Could you check a few things on this model? Use its own coordinates, in mm. A direction names the side the tool comes from. Round coordinates to 2 decimals unless told otherwise and drop trailing zeros. Write each loop counter-clockwise with the first axis right and the second up, starting at its lowest first coordinate (ties: lowest second). Pieces come first, ordered by that corner, then holes. Notation, with made-up numbers: (12.5, 49) -> (41.5, 49) arc R19 cw to (41.5, 67) -> close; hole circle Ø8 at (7.25, 71.25). An arc over 180 degrees is marked (long way). Answer as CSV lines item,"result". Start each with the question number.
Q1. Will these pins go through, and if not, where does the flat tip stop? pin 1 Ø3 at (x, y) = (-23, 2) entering from -Z; pin 2 Ø6 at (x, y) = (-25, 24.5) entering from +Z.
Q2. Imagine slicing it at B-B on z = 42. Please give me the cut outline in (x, y), and give its area (3 significant figures).
Q3. Imagine slicing it at C-C on y = 38. Please give me the cut outline in (x, z).
Q4. If I drill on line 1 (X direction, y = 42, z = 45.5); line 2 (Y direction, x = -59, z = 18); line 3 (Z direction, x = -51.5, y = 20), over which ranges is the centre line in solid material (lowest first)? Write a range as [from, to].
Q5. Imagine slicing it at D-D on y = 16.5. Please give me the cut outline in (x, z).
Q6. If we mould it in two halves opening along X, with no side actions, what happens to faces 1 (the flat face through (-73.66, 16, 19)), 2 (the flat face through (-37, 61.133, 25)), 3 (the flat face through (-37, -11.209, 27))? For each: pulls with the +X half, pulls with the -X half, needs draft (parallel to the pull), parting line crosses it, or undercut.
Q7. Imagine slicing it at A-A on x = -33. Please give me the cut outline in (y, z), and give its area (3 significant figures).
Q8. For faces 4 (the flat face through (-72.493, 24, 16)), 5 (the cylindrical face through (-0.7, 25.75, 43.85)), which set-ups out of +Z, -Z, +X, -X, +Y, -Y let a thin tool reach every point of the face, with its end or its side?
from build123d import *

# Parameters (mm, degrees)
F0_W     = 73.66
F0_H     = 73.66
F1_DEPTH = 50.8
F2_W     = 71.12
F2_H     = 71.12
F3_DEPTH = 48.26
F4_R     = 12.7
F5_DEPTH = 87.376


with BuildPart() as f1:
    # F0 (on Top) → F1 (new body)
    with BuildSketch(Plane.XY):
        with Locations((-36.83, 24.302927)):
            Rectangle(F0_W, F0_H)
    extrude(amount=F1_DEPTH)

    # F2 (on face) → F3 (cut)
    with BuildSketch(Plane.XY.offset(50.8)):
        with Locations((-36.933068, 24.351135)):
            Rectangle(F2_W, F2_H)
    extrude(amount=-F3_DEPTH, mode=Mode.SUBTRACT)

    # F4 (on face) → F5 (cut)
    with BuildSketch(Plane(origin=(-73.66, 0, 0), x_dir=(0, -1, 0), z_dir=(-1, 0, 0))):
        with Locations((-24.100089, 31.257417)):
            Circle(F4_R)
    extrude(amount=-F5_DEPTH, mode=Mode.SUBTRACT)


solid = f1.part
Checks:
1,pin 1,"z = 0"
1,pin 2,"z = 2.54"
2,outline,"(-73.66, -12.53) -> (0, -12.53) -> (0, 17.33) -> (-1.37, 17.33) -> (-1.37, -11.21) -> (-72.49, -11.21) -> (-72.49, 17.33) -> (-73.66, 17.33) -> close; (-73.66, 30.87) -> (-72.49, 30.87) -> (-72.49, 59.91) -> (-1.37, 59.91) -> (-1.37, 30.87) -> (0, 30.87) -> (0, 61.13) -> (-73.66, 61.13) -> close"
2,area,"333 mm^2"
3,outline,"(-73.66, 0) -> (0, 0) -> (0, 50.8) -> (-1.37, 50.8) -> (-1.37, 2.54) -> (-72.49, 2.54) -> (-72.49, 50.8) -> (-73.66, 50.8) -> close"
4,line 1,"[-73.66, -72.49], [-1.37, 0]"
4,line 2,"[-12.53, -11.21], [59.91, 61.13]"
4,line 3,"[0, 2.54]"
5,outline,"(-73.66, 0) -> (0, 0) -> (0, 21.08) -> (-1.37, 21.08) -> (-1.37, 2.54) -> (-72.49, 2.54) -> (-72.49, 21.08) -> (-73.66, 21.08) -> close; (-73.66, 41.43) -> (-72.49, 41.43) -> (-72.49, 50.8) -> (-73.66, 50.8) -> close; (-1.37, 41.43) -> (0, 41.43) -> (0, 50.8) -> (-1.37, 50.8) -> close"
6,face 1,"pulls with the -X half"
6,face 2,"needs draft"
6,face 3,"undercut"
7,outline,"(-12.53, 0) -> (61.13, 0) -> (61.13, 50.8) -> (59.91, 50.8) -> (59.91, 2.54) -> (-11.21, 2.54) -> (-11.21, 50.8) -> (-12.53, 50.8) -> close"
7,area,"310 mm^2"
8,face 4,"+Z"
8,face 5,"+X, -X"
